CAD build for the part. Positions are in the model's coordinates, mm. A direction names the side the tool comes from. Coordinates: 2 decimals unless noted, no trailing zeros. Loops run counter-clockwise (first coordinate to the right, second up) from the corner with the lowest first, then second, coordinate; pieces in that order, holes last. Notation, with made-up numbers: (-10.75, -34.75) -> (41.25, -34.75) arc R17 ccw to (41.25, -6.75) -> close; hole circle Ø8 at (57.5, 7). An arc over 180 degrees is marked (long way). Return JSON: item names as keys, results as strings. Group by question number.
(1) Saw through at C-C on x = -50.5. Write the cut outline in (y, z), then the cut area to 3 significant figures.
(2) Probe L1, parallel to X at y = 8.5, z = -15; L2, parallel to X at y = 9, z = -14; L3, parallel to Y at x = -43.5, z = -4. List the from-to ranges inside material, lowest first.
(3) Flat gauge pins, fed straight in: pin 1 Ø1 at (x, z) = (-27.5, -9) entering from +Y; pin 2 Ø2 at (x, z) = (3.5, 11) entering from +Y; pin 3 Ø6 at (x, z) = (1.5, 7) entering from -Y. Where does each tip first touch, or does it go through?
(4) Saw through at A-A on z = 0. Write the cut outline in (x, y), then the cut area to 3 significant figures.
(5) Tool access for faces 4 (the face through (3, 7.5, -10)), 5 (the face through (-24.795, 22, 0)), 6 (the face through (16, 0, 0)), 7 (the face through (-29, 0, 0)): list every direction of +Z, -Z, +X, -X, +Y, -Y with a clear straight run to the whole face (end or side of a thin tool).
(6) Saw through at B-B on y = -49. Write the cut outline in (x, z).
(7) Mould opens along X. For faces 1 (the face through (-41, 15, 0)), 2 (the face through (-14.795, 22, 0)), 3 (the face through (3, 7.5, 12)) say: pulls with the +X half, pulls with the -X half, needs draft (parallel to the pull), parting line crosses it, or undercut.
```python
from build123d import *

# Parameters (mm, degrees)
SKETCH1_W           = 74
SKETCH1_H           = 15
BOSS_EXTRUDE1_DEPTH = 20
SKETCH2_W           = 10
SKETCH2_H           = 40
BOSS_EXTRUDE2_DEPTH = 30
SKETCH3_R           = 5.024696106
CUT_EXTRUDE4_DEPTH  = 15
SKETCH6_R           = 5
CUT_EXTRUDE5_DEPTH  = 30
SKETCH8_R           = 5
CUT_EXTRUDE6_DEPTH  = 30
SKETCH9_R           = 5
CUT_EXTRUDE7_DEPTH  = 30
SKETCH11_R          = 10
BOSS_EXTRUDE3_DEPTH = 15


with BuildPart() as part:
    # Sketch1 → Boss-Extrude1 (new, symmetric)
    with BuildSketch(Plane.XY):
        with Locations((-19.794871795, 7.5)):
            Rectangle(SKETCH1_W, SKETCH1_H)
    extrude(amount=BOSS_EXTRUDE1_DEPTH, both=True)

    # Sketch2 → Boss-Extrude2 (add)
    with BuildSketch(Plane(origin=(0, 0, 0), x_dir=(1, 0, 0), z_dir=(0, 1, 0))):
        with Locations((-19.794871795, 0)):
            Rectangle(SKETCH2_W, SKETCH2_H)
    extrude(amount=BOSS_EXTRUDE2_DEPTH)

    # Sketch3 → Cut-Extrude4 (cut)
    with BuildSketch(Plane(origin=(0, 0, 0), x_dir=(1, 0, 0), z_dir=(0, 1, 0))):
        with Locations(Location((-41.794871795, 11.238480193, 0), (0, 0, 90))):
            Circle(SKETCH3_R)
    extrude(amount=CUT_EXTRUDE4_DEPTH, mode=Mode.SUBTRACT)

    # Sketch6 → Cut-Extrude5 (cut)
    with BuildSketch(Plane(origin=(0, 15, 0), x_dir=(1, 0, 0), z_dir=(0, 1, 0))):
        with Locations(Location((-41.794871795, -7.874935053, 0), (0, 0, 270))):
            Circle(SKETCH6_R)
    extrude(amount=-CUT_EXTRUDE5_DEPTH, mode=Mode.SUBTRACT)

    # Sketch8 → Cut-Extrude6 (cut)
    with BuildSketch(Plane(origin=(0, 15, 0), x_dir=(1, 0, 0), z_dir=(0, 1, 0))):
        with Locations(Location((2.205128205, 10.435706621, 0), (0, 0, 270))):
            Circle(SKETCH8_R)
    extrude(amount=-CUT_EXTRUDE6_DEPTH, mode=Mode.SUBTRACT)

    # Sketch9 → Cut-Extrude7 (cut)
    with BuildSketch(Plane(origin=(0, 15, 0), x_dir=(1, 0, 0), z_dir=(0, 1, 0))):
        with Locations(Location((2.205128205, -11.598088542, 0), (0, 0, 270))):
            Circle(SKETCH9_R)
    extrude(amount=-CUT_EXTRUDE7_DEPTH, mode=Mode.SUBTRACT)

    # Sketch11 → Boss-Extrude3 (add)
    with BuildSketch(Plane(origin=(0, 0, 0), x_dir=(0, 0, -1), z_dir=(1, 0, 0))):
        with BuildLine():
            Line((-20, 7.5), (20, 7.5))
            Line((20, 7.5), (20, -42.5))
            ThreePointArc((20, -42.5), (0, -62.270254711), (-20, -42.5))
            Line((-20, -42.5), (-20, 7.5))
        make_face()
        with Locations((0, -42.268919804)):
            Circle(SKETCH11_R, mode=Mode.SUBTRACT)
    extrude(amount=BOSS_EXTRUDE3_DEPTH)


solid = part.part
```
Geometry results:
{
 "1": {"outline": "(0, -20) -> (15, -20) -> (15, 20) -> (0, 20) -> close", "area": "600 mm²"},
 "2": {"L1": "-56.79 to -45.13, -38.46 to 0.16, 4.25 to 17.21", "L2": "-56.79 to -45.99, -37.6 to -1.3, 5.71 to 17.21", "L3": "0 to 15"},
 "3": {"pin 1": "y = 15", "pin 2": "y = 7.5", "pin 3": "y = -61.87"},
 "4": {"outline": "(-56.79, 0) -> (0, 0) -> (0, -32.27) -> (15, -32.27) -> (15, 0) -> (17.21, 0) -> (17.21, 15) -> (-14.79, 15) -> (-14.79, 30) -> (-24.79, 30) -> (-24.79, 15) -> (-56.79, 15) -> close; (0, -62.27) -> (15, -62.27) -> (15, -52.27) -> (0, -52.27) -> close", "area": "1,890 mm²"},
 "5": {"face 4": "+Y", "face 5": "+Z, -Z, -X, +Y", "face 6": "+Z, -Z, +X, -Y", "face 7": "+Z, -Z, -X, -Y"},
 "6": {"outline": "(0, -18.83) -> (15, -18.83) -> (15, -7.4) -> (0, -7.4) -> close; (0, 7.4) -> (15, 7.4) -> (15, 18.83) -> (0, 18.83) -> close"},
 "7": {"face 1": "needs draft", "face 2": "pulls with the +X half", "face 3": "undercut"}
}
